Autodesk Inventor part; units mm, degrees
ref_plane "Start Plane" through (0, 0, 0) normal (0, 0, 1) x (1, 0, 0)
ref_plane "End Plane" through (0, 0, 700) normal (0, 0, 1) x (1, 0, 0)
ref_plane "YZ Plane" through (0, 0, 0) normal (1, 0, 0) x (0, 1, 0)
ref_plane "Start Plane" through (0, 0, 0) normal (0, 0, 1) x (1, 0, 0)
ref_plane "End Plane" through (0, 0, 700) normal (0, 0, 1) x (1, 0, 0)
sketch "Sketch" plane through (0, 0, 0) normal (0, 0, 1) x (1, 0, 0)
  line L0 (-20, -16) -> (-20, 16)
  line L1 (-16, 20) -> (16, 20)
  line L2 (20, 16) -> (20, -16)
  line L3 (16, -20) -> (-16, -20)
  arc A0 (-20, -16) -> (-16, -20) centre (-16, -16) ccw
  arc A1 (20, 16) -> (16, 20) centre (16, 16) ccw
  arc A2 (-16, 20) -> (-20, 16) centre (-16, 16) ccw
  arc A3 (16, -20) -> (20, -16) centre (16, -16) ccw
  arc A4 (-16, 18) -> (-18, 16) centre (-16, 16) ccw
  line L4 (-16, 18) -> (16, 18)
  arc A5 (18, 16) -> (16, 18) centre (16, 16) ccw
  line L5 (18, 16) -> (18, -16)
  arc A6 (16, -18) -> (18, -16) centre (16, -16) ccw
  line L6 (16, -18) -> (-16, -18)
  arc A7 (-18, -16) -> (-16, -18) centre (-16, -16) ccw
  line L7 (-18, -16) -> (-18, 16)
  line L8 (0, 29.1598) -> (0, -29.1598) construction
  line L9 (-29.1598, 0) -> (29.1598, 0) construction
  dimension "d7" = 4
  dimension "d9" = 40
  dimension "d11" = 40
  dimension "d12" = 2
  dimension "d15" = 20
  dimension "d16" = 20
extrude "Body" add sketch "Sketch" along normal up to surface (700 mm away) from surface at 0
sketch "Sketch3" plane through (0, 0, 0) normal (0, 0, 1) x (1, 0, 0)
  line L0 (0, 0) -> (10, 0)
ref_plane "Work Plane3" through (0, 0, 0) normal (0, -1, 0) x (1, 0, 0)
sketch "Sketch5" plane through (16, 20, 700) normal (0, 1, 0) x (1, 0, 0)
  line L0 (-32, 0) -> (0, 0) construction
  line L1 (0, 700) -> (0, 0) construction
  line L2 (-32, 700) -> (0, 700)
  line L3 (-32, 700) -> (-32, 0) construction
  circle A0 centre (-16, 40) radius 5.5
  circle A1 centre (-16, 240) radius 5.5
  point P0 (-16, 700)
  point P1 (-16, 0)
  dimension "d19" = 11
  dimension "d20" = 40
  dimension "d21" = 200
extrude "Extrusion2" cut sketch "Sketch5" against normal up to surface (2 mm away)
sketch "Sketch4" plane through (0, 0, 0) normal (0, -1, 0) x (1, 0, 0)
  line L0 (-2, 0) -> (12, 0)
  line L1 (-2, 700) -> (12, 700)
  dimension "d18" = 700
equation "\"d7\" = G_IR"
equation "\"d9\" = G_W"
equation "\"d11\" = G_H"
equation "\"d12\" = G_T"
equation "\"d15\" = 0.5 * d9"
equation "\"d16\" = 0.5 * d11"
equation "\"d3\" = G_L"
equation "\"G_W\" = 40"
equation "\"G_H\" = 40"
equation "\"G_T\" = 2"
equation "\"G_IR\" = 4"
equation "\"G_L\" = d18"
equation "\"G_OFFSET_START\" = 0"
equation "\"G_OFFSET_END\" = 0"
properties part number "ISO 10799-2 40x40x2 1714907750312" material "Stainless Steel"
Work out the finished part from the listing and answer in its coordinate system (mm). A direction names the side the tool comes from. Give positions to 0.01 mm unless a question says otherwise; leave off trailing zeros. Loops run counter-clockwise (first coordinate to the right, second up) from the corner with the lowest first, then second, coordinate; pieces in that order, holes last. Notation, with made-up numbers: (71.25, 15.25) - (104.25, 15.25) arc R12 ccw to (104.25, 34.25) - close; hole circle Ø6 at (-5, 34). An arc over 180 degrees is marked (long way). Use CSV: the item, a comma, the result in double quotes. Start each with the question number.
(1) Find section A-A, the plane y = 8. Determine the outline of the cut face in (x, z), plus the area to 3 significant figures.
(2) Find the intervals of material crossed by L1, parallel to Z at x = 0, y = 19; L2, parallel to X at y = 13.5, z = 601; L3, parallel to X at y = -16.5, z = 519, in increasing order.
(3) This flat-tipped pin is pushed along its axis until it touches: pin 1 (17.5 mm diameter, centred on x = 0, z = 660, fed in from +Y). Where does it stop, or does it pass through?
(4) Determine the mould class of faces 4 (the face through (-2, -19, 0)), 5 (the face through (-4.05, 19.01, 656.28)), 6 (the face through (-20, 0, 345)), 7 (the face through (-18, 0, 345)) for opening direction X: released by +X, released by -X, zero draft, split by the parting line, or undercut.
(5) A tool of negligible diameter and unlimited length cuts with its end or side. For faces 1 (the face through (20, 0, 345)), 2 (the face through (-1.19, 19.01, 465.37)), 3 (the face through (0, 18, 345)), from which of +Z, -Z, +X, -X, +Y, -Y can it reach the whole face along a straight path? Write none if from no direction.
(6) Find section B-B, the plane z = 647.5. Determine the outline of the cut face in (x, y).
Results found:
1,outline,"(-20, 0) - (-18, 0) - (-18, 700) - (-20, 700) - close; (18, 0) - (20, 0) - (20, 700) - (18, 700) - close"
1,area,"2,800 mm^2"
2,L1,"0 to 454.5, 465.5 to 654.5, 665.5 to 700"
2,L2,"-20 to -18, 18 to 20"
2,L3,"-19.97 to -17.94, 17.94 to 19.97"
3,pin 1,"y = 20"
4,face 4,"zero draft"
4,face 5,"undercut"
4,face 6,"released by -X"
4,face 7,"undercut"
5,face 1,"+Z, -Z, +X, +Y, -Y"
5,face 2,"+Y"
5,face 3,"+Z, -Z"
6,outline,"(-20, -16) arc R4 ccw to (-16, -20) - (16, -20) arc R4 ccw to (20, -16) - (20, 16) arc R4 ccw to (16, 20) - (-16, 20) arc R4 ccw to (-20, 16) - close; hole (-18, -16) arc R2 ccw to (-16, -18) - (16, -18) arc R2 ccw to (18, -16) - (18, 16) arc R2 ccw to (16, 18) - (-16, 18) arc R2 ccw to (-18, 16) - close"
